For this review, take the finished solid that the model builds, in its own axes (mm). A direction names the side the tool comes from. Round coordinates to 2 decimals unless told otherwise and drop trailing zeros. Loops run counter-clockwise (first coordinate to the right, second up) from the corner with the lowest first, then second, coordinate; pieces in that order, holes last. Notation, with made-up numbers: (58, 39.5) -> (73, 39.5) arc R28 ccw to (73, 63.5) -> close; hole circle Ø2 at (75, 23.25). An arc over 180 degrees is marked (long way). One line per question, with ' | ' between items. Start each with the question number.
1. Consider section B-B (x = 0). Write out the cut boundary in (y, z), and give its area (4 significant figures).
2. Draft analysis for pull direction Y (two halves, no side actions). For faces 1 (the face through (-9.496, 0.259, 1.972)), 2 (the face through (-3, 0, 0)), 3 (the face through (-5.497, 0.174, 2.768)), 4 (the face through (-0.596, -2.685, 0.74)), state which applies: pulls with the +Y half, pulls with the -Y half, needs draft (parallel to the pull), parting line crosses it, or undercut.
3. Consider section D-D (z = 2.65). Write out the cut boundary in (x, y).
4. Wall thickness on line 1 along Y through (x, z) = (0, 0.7); line 2 along Y through (x, z) = (1.75, 2.3); line 3 along Z through (x, y) = (-2, 4.5): over which ranges is each line inside the solid? List them lowest first.
5. For faces 5 (the face through (-6, -2, 4)), 6 (the face through (-3, 0, 1.5)), list the 3-axis set-ups (+Z, -Z, +X, -X, +Y, -Y) from which the entire face can be reached by the end or side of a thin tool; tool diameter is ignored.
6. Consider section C-C (y = -2.5). Write out the cut boundary in (x, z), and give its area (3 significant figures).
7. Consider section A-A (y = 0). Write out the cut boundary in (x, z).
8. For pin 1 Ø2 at (x, y) = (-7.5, 3.5) entering from -Z; pin 2 Ø4.5 at (x, y) = (0.5, 2.5) entering from +Z, all flat-tipped, find the tip position at first contact; note any pin that passes through.
```python
from build123d import *

# Parameters (mm, degrees)
ESQUISSE1_R             = 9.5
ESQUISSE1_R_2           = 2.75
ESQUISSE1_R_3           = 1.5
BOSS_EXTRU_1_DEPTH      = 4
ESQUISSE2_W             = 6
ESQUISSE2_H             = 17.663521732
ENL_V_MAT_EXTRU_1_DEPTH = 15.017845769
ESQUISSE3_R             = 5.5
ENL_V_MAT_EXTRU_2_DEPTH = 2.5


with BuildPart() as part:
    # Esquisse1 → Boss.-Extru.1 (new body)
    with BuildSketch(Plane.XY):
        Circle(ESQUISSE1_R)
        Circle(ESQUISSE1_R_2, mode=Mode.SUBTRACT)
        with Locations((-7.5, 0)):
            Circle(ESQUISSE1_R_3, mode=Mode.SUBTRACT)
    extrude(amount=BOSS_EXTRU_1_DEPTH)

    # Esquisse2 → Enlèv. mat.-Extru.1 (cut, through all)
    with BuildSketch(Plane.XY.offset(4)):
        with Locations((6.5, 0)):
            Rectangle(ESQUISSE2_W, ESQUISSE2_H)
    extrude(amount=-ENL_V_MAT_EXTRU_1_DEPTH, mode=Mode.SUBTRACT)

    # Esquisse3 → Enlèv. mat.-Extru.2 (cut)
    with BuildSketch(Plane.XY.offset(4)):
        Circle(ESQUISSE3_R)
    extrude(amount=-ENL_V_MAT_EXTRU_2_DEPTH, mode=Mode.SUBTRACT)


solid = part.part
```
Answer block:
1) outline: (-9.5, 0) -> (-2.75, 0) -> (-2.75, 1.5) -> (-5.5, 1.5) -> (-5.5, 4) -> (-9.5, 4) -> close; (2.75, 0) -> (9.5, 0) -> (9.5, 4) -> (5.5, 4) -> (5.5, 1.5) -> (2.75, 1.5) -> close | area: 40.25 mm2
2) face 1: parting line crosses it | face 2: needs draft | face 3: undercut | face 4: undercut
3) outline: (3.5, -8.83) -> (3.5, -4.24) arc R5.5 cw (long way) to (3.5, 4.24) -> (3.5, 8.83) arc R9.5 ccw (long way) to start; hole circle Ø3 at (-7.5, 0)
4) line 1: y = -9.5 to -2.75, 2.75 to 9.5 | line 2: y = -9.34 to -5.21, 5.21 to 9.34 | line 3: z = 0 to 1.5
5) face 5: +Z, +X, -X, +Y, -Y | face 6: +Z
6) outline: (-9.17, 0) -> (-1.15, 0) -> (-1.15, 1.5) -> (-4.9, 1.5) -> (-4.9, 4) -> (-9.17, 4) -> close; (1.15, 0) -> (3.5, 0) -> (3.5, 1.5) -> (1.15, 1.5) -> close | area: 26.2 mm2
7) outline: (-9.5, 0) -> (-9, 0) -> (-9, 4) -> (-9.5, 4) -> close; (-6, 0) -> (-2.75, 0) -> (-2.75, 1.5) -> (-5.5, 1.5) -> (-5.5, 4) -> (-6, 4) -> close; (2.75, 0) -> (3.5, 0) -> (3.5, 1.5) -> (2.75, 1.5) -> close
8) pin 1: stops at z = 0 | pin 2: stops at z = 1.5
